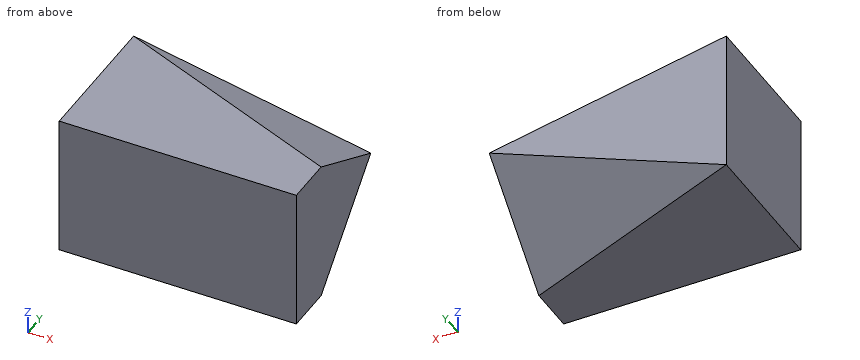
Autodesk Inventor part; units mm, degrees
ref_plane "工作平面1" through (0, 30, 0) normal (0.1761, 0.4402, 0.8805) x (0.9285, -0.3714, 0)
ref_plane "工作平面2" through (0, 30, -30) normal (0.2722, 0.6804, -0.6804) x (0.9285, 0, 0.3714)
ref_plane "YZ Plane" through (0, 0, 0) normal (1, 0, 0) x (0, 1, 0)
sketch "草圖1" plane through (0, 0, 0) normal (0, 1, 0) x (-1, 0, 0)
  line L0 (0, 0) -> (-50, 0)
  line L1 (-50, 0) -> (-50, -30)
  line L2 (-50, -30) -> (0, -30)
  line L3 (0, -30) -> (0, 0)
  dimension "d0" = 30
  dimension "d1" = 50
extrude "擠出1" add sketch "草圖1" along normal blind 30
sketch "草圖2" plane through (50, 0, 0) normal (1, 0, 0) x (0, 0, -1)
  line L0 (0, 0) -> (0, 30)
  line L1 (0, 10) -> (10, 30)
  line L2 (0, 30) -> (30, 30)
  dimension "d4" = 10
  dimension "d5" = 20
ref_plane "工作平面1" through (0, 30, 0) normal (0.1761, 0.4402, 0.8805) x (0.9285, -0.3714, 0)
sketch "草圖3" plane through (0, 30, 0) normal (0.1761, 0.4402, 0.8805) x (0.9285, -0.3714, 0)
  line L0 (-15.4491, 27.3305) -> (88.7028, 27.3305)
  line L1 (88.7028, 27.3305) -> (88.7028, -20.9863)
  line L2 (88.7028, -20.9863) -> (-15.4491, -20.9863)
  line L3 (-15.4491, -20.9863) -> (-15.4491, 27.3305)
  point P0 (11.1417, -24.5243)
extrude "擠出2" cut sketch "草圖3" along normal blind 30
sketch "草圖4" plane through (50, 0, 0) normal (1, 0, 0) x (0, 0, -1)
  line L0 (30, 0) -> (30, 30)
  point P0 (0, 0)
  point P1 (30, 10)
  dimension "d8" = 20
ref_plane "工作平面2" through (0, 30, -30) normal (0.2722, 0.6804, -0.6804) x (0.9285, 0, 0.3714)
sketch "草圖5" plane through (0, 30, -30) normal (0.2722, 0.6804, -0.6804) x (0.9285, 0, 0.3714)
  line L0 (63.1624, -12.2255) -> (-24.2943, -12.2255)
  line L1 (-24.2943, -12.2255) -> (-24.2943, 28.5728)
  line L2 (-24.2943, 28.5728) -> (63.1624, 28.5728)
  line L3 (63.1624, 28.5728) -> (63.1624, -12.2255)
  point P0 (11.1417, 3.0324)
extrude "擠出3" cut sketch "草圖5" along normal blind 30
properties part number "40"
The listing builds one solid part. Answer for the finished solid, in the listing's coordinates (mm). Coordinates: 2 decimals unless noted, no trailing zeros. Write each loop counter-clockwise with the first axis right and the second up, starting at its lowest first coordinate (ties: lowest second). Pieces come first, ordered by that corner, then holes. Notation, with made-up numbers: (-14, 8.25) -> (5, 8.25) arc R18 ccw to (5, 40.25) -> close; hole circle Ø6 at (8, 57). An arc over 180 degrees is marked (long way). Write each question's results on one line, items separated by ' | '. Start each with the question number.
1) Straight lines are drawn through the part: probe 1 along X at (y, z) = (17, -29); probe 2 along Z at (x, y) = (25, 28); probe 3 along Y at (x, z) = (33.5, -22). For each, find the intervals that lie inside material, in ascending order.
2) A cutting plane is placed at B-B (x = 16). Determine the outline of the cut face in (y, z), then the cut area to 3 significant figures.
3) Flat-ended cylindrical pins translate along their axes: pin 1 Ø2 at (x, z) = (23, -25) entering from +Y; pin 2 Ø2 at (x, z) = (17.5, -19) entering from -Y. Find the tip coordinate at first contact, or state that the pin passes through.
4) A cutting plane is placed at C-C (z = -22). Determine the outline of the cut face in (x, y).
5) A cutting plane is placed at D-D (z = -14.5). Determine the outline of the cut face in (x, y), then the cut area to 3 significant figures.
6) A cutting plane is placed at A-A (y = 18). Determine the outline of the cut face in (x, z).
Values follow:
1) probe 1: 0 to 34.99 | probe 2: -22 to -4 | probe 3: 0 to 24.6
2) outline: (0, -30) -> (23.6, -30) -> (30, -23.6) -> (30, -3.2) -> (23.59, 0) -> (0, 0) -> close | area: 869 mm²
3) pin 1: y = 26.87 | pin 2: y = 0
4) outline: (0, 0) -> (50, 0) -> (50, 17.99) -> (19.99, 30) -> (0, 30) -> close
5) outline: (0, 0) -> (50, 0) -> (50, 25.49) -> (38.74, 30) -> (0, 30) -> close | area: 1,470 mm²
6) outline: (0, -30) -> (29.99, -30) -> (50, -21.99) -> (50, -4) -> (29.99, 0) -> (0, 0) -> close
